Could you check a few things on this drawing? It's one solid part, dimensions in mm from its lowest x, y, z. A direction names the side the tool comes from. Give positions to 0.01 mm unless a question says otherwise; leave off trailing zeros. Write each loop counter-clockwise with the first axis right and the second up, starting at its lowest first coordinate (ties: lowest second). Pieces come first, ordered by that corner, then holes.
1. Thinking about a two-plate mould opening in X: for the marked faces 3, 4 and 5, which applies, pulls with the +X half, pulls with the -X half, needs draft (parallel to the pull), parting line crosses it, or undercut?
2. On a 3-axis mill with a long thin cutter (end or side, diameter ignored), from which of +Z, -Z, +X, -X, +Y, -Y can I reach the whole of each face in a straight line? I mean the marked faces 1 and 2. Say none if no direction works.
3. I'm going to push a flat-ended pin straight in: pin 1 (6.5 mm diameter, centred on x = 33, y = 6, fed in from -Z). Where does the tip first touch, or does it pass through?
4. If I drill on probe 1 along X at (y, z) = (10, 0.75); probe 2 along Z at (x, y) = (30.5, 11); probe 3 along X at (y, z) = (7.25, 5.25), over which ranges is the centre line in solid material (lowest first)?
5. Suppose I cut it at C-C (x = 29). Please give me the cut outline in (y, z), and give its area (3 significant figures).
6. Suppose I cut it at B-B (z = 4.25). Please give me the cut outline in (x, y), and give its area (3 significant figures).
7. Suppose I cut it at A-A (y = 8.5). Please give me the cut outline in (x, z), and give its area (3 significant figures).
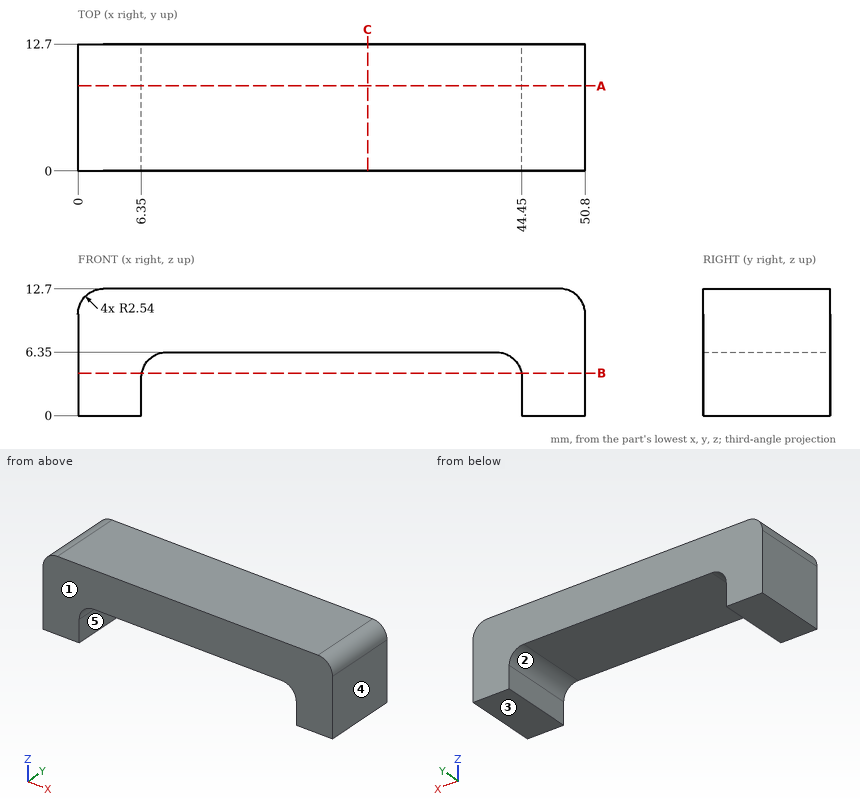
Checks:
1. face 3: needs draft
1. face 4: pulls with the +X half
1. face 5: undercut
2. face 1: +Z, -Z, +X, -X, -Y
2. face 2: -Z, +Y, -Y
3. pin 1: stops at z = 6.35
4. probe 1: x = 0 to 6.35, 44.45 to 50.8
4. probe 2: z = 6.35 to 12.7
4. probe 3: x = 0 to 6.8, 44 to 50.8
5. outline: (0, 6.35) - (12.7, 6.35) - (12.7, 12.7) - (0, 12.7) - close
5. area: 80.6 mm2
6. outline: (0, 0) - (6.39, 0) - (6.39, 12.7) - (0, 12.7) - close; (44.41, 0) - (50.8, 0) - (50.8, 12.7) - (44.41, 12.7) - close
6. area: 162 mm2
7. outline: (0, 0) - (6.35, 0) - (6.35, 3.81) arc R2.54 cw to (8.89, 6.35) - (41.91, 6.35) arc R2.54 cw to (44.45, 3.81) - (44.45, 0) - (50.8, 0) - (50.8, 10.16) arc R2.54 ccw to (48.26, 12.7) - (2.54, 12.7) arc R2.54 ccw to (0, 10.16) - close
7. area: 403 mm2
